```python
from build123d import *

# Parameters (mm, degrees)
EXTRUDE_1_DEPTH     = 20
CUT_EXTRUDE_1_REACH = 5
SKETCH_2_R          = 8
CUT_EXTRUDE_2_REACH = 5
SKETCH_3_R          = 1.5
SKETCH_6_W          = 20
SKETCH_6_H          = 3
EXTRUDE_2_DEPTH     = 5
SKETCH_8_W          = 20
SKETCH_8_H          = 27
CUT_EXTRUDE_5_DEPTH = 1
SKETCH_10_W         = 20
SKETCH_10_H         = 3
CUT_EXTRUDE_7_DEPTH = 18
SKETCH_11_W         = 20
SKETCH_11_H         = 18
CUT_EXTRUDE_8_DEPTH = 1
SKETCH_12_R         = 1.5
CUT_EXTRUDE_9_DEPTH = 2


with BuildPart() as part:
    # 草图1 → 凸台-拉伸1 (new body)
    with BuildSketch(Plane(origin=(0, 0, 0), x_dir=(0, 0, -1), z_dir=(1, 0, 0))):
        Polygon((0, 0), (0, 22), (3, 22), (3, -3), (-35, -3), (-35, 0), align=None)
    extrude(amount=EXTRUDE_1_DEPTH)

    # 草图2 → 切除-拉伸1 (cut, up to next)
    with BuildSketch(Plane.XY, mode=Mode.PRIVATE) as cut_extrude_1_sk1:
        with Locations((10, 13)):
            Circle(SKETCH_2_R)
    cut_extrude_1_tool1 = extrude(cut_extrude_1_sk1.sketch, amount=-CUT_EXTRUDE_1_REACH, mode=Mode.PRIVATE) & part.part
    add(cut_extrude_1_tool1.solids().sort_by_distance((10, 13, 0))[0], mode=Mode.SUBTRACT)

    # 草图3 → 切除-拉伸2 (cut, up to next)
    with BuildSketch(Plane(origin=(0, 0, 0), x_dir=(1, 0, 0), z_dir=(0, 1, 0)), mode=Mode.PRIVATE) as cut_extrude_2_sk1:
        with Locations((4, -4)):
            Circle(SKETCH_3_R)
    cut_extrude_2_tool1 = extrude(cut_extrude_2_sk1.sketch, amount=-CUT_EXTRUDE_2_REACH, mode=Mode.PRIVATE) & part.part
    add(cut_extrude_2_tool1.solids().sort_by_distance((4, 0, 4))[0], mode=Mode.SUBTRACT)
    # 草图3 → 切除-拉伸2 (cut, up to next)
    with BuildSketch(Plane(origin=(0, 0, 0), x_dir=(1, 0, 0), z_dir=(0, 1, 0)), mode=Mode.PRIVATE) as cut_extrude_2_sk2:
        with Locations((16, -4)):
            Circle(SKETCH_3_R)
    cut_extrude_2_tool2 = extrude(cut_extrude_2_sk2.sketch, amount=-CUT_EXTRUDE_2_REACH, mode=Mode.PRIVATE) & part.part
    add(cut_extrude_2_tool2.solids().sort_by_distance((16, 0, 4))[0], mode=Mode.SUBTRACT)

    # 草图6 → 凸台-拉伸2 (add)
    with BuildSketch(Plane(origin=(0, 22, 0), x_dir=(1, 0, 0), z_dir=(0, 1, 0))):
        with Locations((10, 1.5)):
            Rectangle(SKETCH_6_W, SKETCH_6_H)
    extrude(amount=EXTRUDE_2_DEPTH)

    # 草图8 → 切除-拉伸5 (cut)
    with BuildSketch(Plane.XY):
        with Locations((10, 13.5)):
            Rectangle(SKETCH_8_W, SKETCH_8_H)
    extrude(amount=-CUT_EXTRUDE_5_DEPTH, mode=Mode.SUBTRACT)

    # 草图10 → 切除-拉伸7 (cut)
    with BuildSketch(Plane.XY.offset(35)):
        with Locations((10, -1.5)):
            Rectangle(SKETCH_10_W, SKETCH_10_H)
    extrude(amount=-CUT_EXTRUDE_7_DEPTH, mode=Mode.SUBTRACT)

    # 草图11 → 切除-拉伸8 (cut)
    with BuildSketch(Plane(origin=(0, 0, 0), x_dir=(1, 0, 0), z_dir=(0, 1, 0))):
        with Locations((10, -8)):
            Rectangle(SKETCH_11_W, SKETCH_11_H)
    extrude(amount=-CUT_EXTRUDE_8_DEPTH, mode=Mode.SUBTRACT)

    # 草图12 → 切除-拉伸9 (cut)
    with BuildSketch(Plane(origin=(0, -1, 0), x_dir=(1, 0, 0), z_dir=(0, 1, 0))):
        with Locations((4, -14)):
            Circle(SKETCH_12_R)
        with Locations((16, -14)):
            Circle(SKETCH_12_R)
    extrude(amount=-CUT_EXTRUDE_9_DEPTH, mode=Mode.SUBTRACT)


solid = part.part
```
The listing builds one solid part. Answer for the finished solid, in the listing's coordinates (mm). A direction names the side the tool comes from. Coordinates: 2 decimals unless noted, no trailing zeros. Write each loop counter-clockwise with the first axis right and the second up, starting at its lowest first coordinate (ties: lowest second). Pieces come first, ordered by that corner, then holes. Notation, with made-up numbers: (-30.5, -2.75) - (9.5, -2.75) arc R16 ccw to (9.5, 24.25) - close; hole circle Ø4 at (26, 35). An arc over 180 degrees is marked (long way). Return JSON: item names as keys, results as strings. Group by question number.
Q1. The part is cut by section B-B on y = 13. Write down the section's boundary in (x, z).
Q2. Which of the six approach directions +Z, -Z, +X, -X, +Y, -Y give full straight-line access (tool end or side, diameter ignored) to faces 5 (the flat face through (1, 13, -1)), 6 (the cylindrical face through (14.5, -1.99, 3.93))?
Q3. For a pull along X with two mould halves and no side action, classify faces 1 (the cylindrical face through (14.5, -1.99, 13.93)), 2 (the flat face through (20, 6, -2)), 3 (the cylindrical face through (5.386, -1.986, 14.575)), 4 (the flat face through (0, 6, -2)) as +X half, -X half, draft (parallel to the pull), parting line (faces both ways), or undercut.
Q4. Flat-ended cylindrical pins translate along their axes: pin 1 Ø3 at (x, y) = (3.5, 15.5) entering from +Z; pin 2 Ø3.5 at (x, z) = (16, 14) entering from -Y; pin 3 Ø2 at (x, z) = (11, 5) entering from +Y. Find the tip coordinate at first contact, or state that the pin passes through.
Q5. The part is cut by section A-A on x = 10. Write down the section's boundary in (y, z).
Q6. Find the intervals of material crossed by line 1 along X through (y, z) = (-2.5, 4); line 2 along Z through (x, y) = (16, -2.15); line 3 along Y through (x, z) = (16.75, 2.5), in increasing order. Write a range as [from, to].
Q7. The part is cut by section D-D on x = 16. Write down the section's boundary in (y, z).
Q8. The part is cut by section C-C on z = 4. Write down the section's boundary in (x, y).
Evaluation:
{
 "1": {"outline": "(0, -3) - (2, -3) - (2, -1) - (0, -1) - close; (18, -3) - (20, -3) - (20, -1) - (18, -1) - close"},
 "2": {"face 5": "+Z, +X, -X, +Y", "face 6": "+Y, -Y"},
 "3": {"face 1": "undercut", "face 2": "+X half", "face 3": "undercut", "face 4": "-X half"},
 "4": {"pin 1": "stops at z = -1", "pin 2": "stops at y = -3", "pin 3": "stops at y = -1"},
 "5": {"outline": "(-3, -3) - (5, -3) - (5, -1) - (-1, -1) - (-1, 17) - (-3, 17) - close; (21, -3) - (27, -3) - (27, -1) - (21, -1) - close"},
 "6": {"line 1": "x = [0, 2.5], [5.5, 14.5], [17.5, 20]", "line 2": "z = [-3, 2.5], [5.5, 12.5], [15.5, 17]", "line 3": "y = [-3, -1]"},
 "7": {"outline": "(-3, -3) - (7.71, -3) - (7.71, -1) - (-1, -1) - (-1, 2.5) - (-3, 2.5) - close; (-3, 5.5) - (-1, 5.5) - (-1, 12.5) - (-3, 12.5) - close; (-3, 15.5) - (-1, 15.5) - (-1, 17) - (-3, 17) - close; (18.29, -3) - (27, -3) - (27, -1) - (18.29, -1) - close"},
 "8": {"outline": "(0, -3) - (2.5, -3) - (2.5, -1) - (0, -1) - close; (5.5, -3) - (14.5, -3) - (14.5, -1) - (5.5, -1) - close; (17.5, -3) - (20, -3) - (20, -1) - (17.5, -1) - close"}
}
